Can you work these out from the drawing? Everything is in mm from the part's minimum corner. A direction names the side the tool comes from. Round coordinates to 2 decimals unless told otherwise and drop trailing zeros. Loops run counter-clockwise (first coordinate to the right, second up) from the corner with the lowest first, then second, coordinate; pieces in that order, holes last. Notation, with made-up numbers: M 10,1.5 L 51,1.5 A14 cw 51,9.5 Z; hole C 79,65.5 d8. An arc over 180 degrees is marked long. Use a Markdown table: item, result.
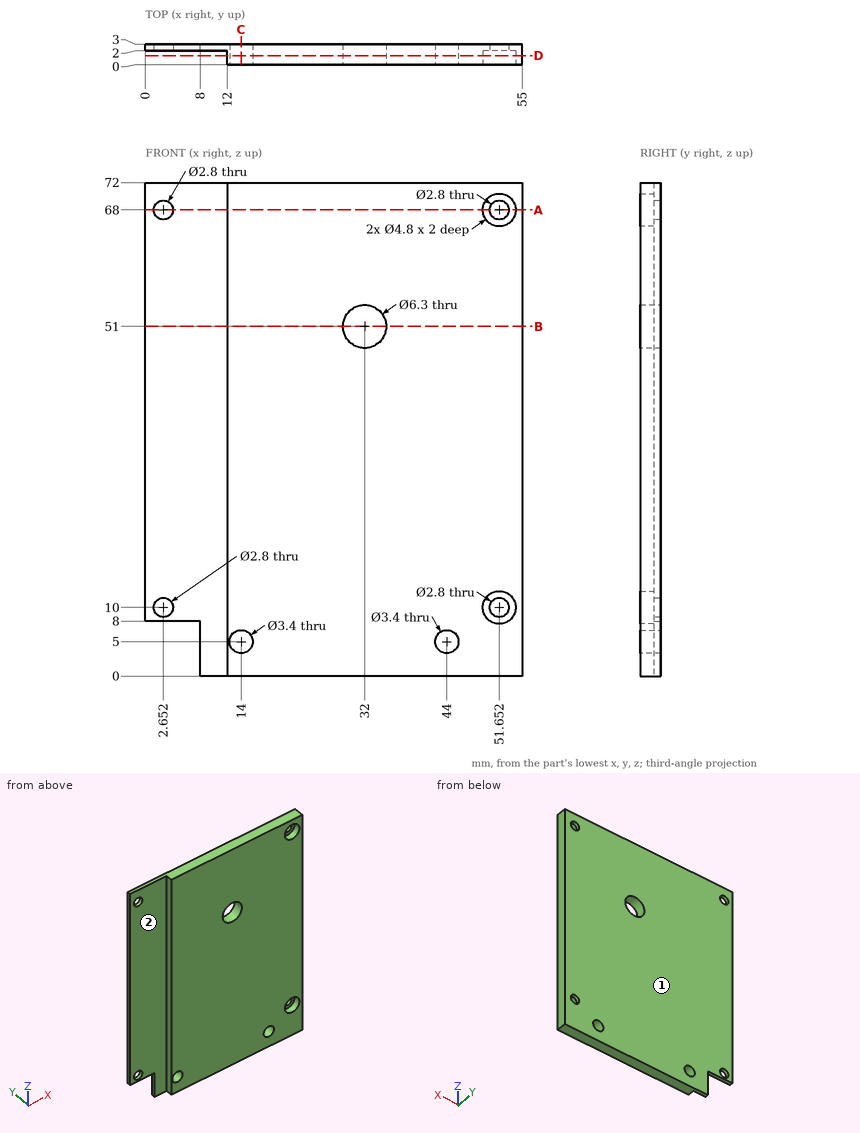
1. Imagine slicing it at A-A, the plane z = 68. Write out the boundary of the cut face in (x, y).
Answer sheet:
| item | result |
|---|---|
| outline | M 0,2 L 1.25,2 L 1.25,3 L 0,3 Z; M 4.05,2 L 12,2 L 12,0 L 49.25,0 L 49.25,2 L 50.25,2 L 50.25,3 L 4.05,3 Z; M 53.05,2 L 54.05,2 L 54.05,0 L 55,0 L 55,3 L 53.05,3 Z |
2. Imagine slicing it at B-B, the plane z = 51. Write out the boundary of the cut face in (x, y), then the cut area to 3 significant figures.
Answer sheet:
| item | result |
|---|---|
| outline | M 0,2 L 12,2 L 12,0 L 28.85,0 L 28.85,3 L 0,3 Z; M 35.15,0 L 55,0 L 55,3 L 35.15,3 Z |
| area | 122 mm2 |
3. Imagine slicing it at C-C, the plane x = 14. Write out the boundary of the cut face in (y, z), then the cut area to 3 significant figures.
Answer sheet:
| item | result |
|---|---|
| outline | M 0,0 L 3,0 L 3,3.3 L 0,3.3 Z; M 0,6.7 L 3,6.7 L 3,72 L 0,72 Z |
| area | 206 mm2 |
4. I need wall thicknesses on probe 1 along X at (y, z) = (2.5, 68); probe 2 along Y at (x, z) = (8.5, 6.5); probe 3 along X at (y, z) = (1, 35). Which ranges of each line are inside material? Lowest first, please. Write a range as from..to.
Answer sheet:
| item | result |
|---|---|
| probe 1 | 0..1.25, 4.05..50.25, 53.05..55 |
| probe 2 | 2..3 |
| probe 3 | 12..55 |
5. Imagine slicing it at D-D, the plane y = 1.3. Write out the boundary of the cut face in (x, z).
Answer sheet:
| item | result |
|---|---|
| outline | M 12,0 L 55,0 L 55,72 L 12,72 Z; hole C 14,5 d3.4; hole C 32,51 d6.3; hole C 44,5 d3.4; hole C 51.65,10 d4.8; hole C 51.65,68 d4.8 |
6. Which directions (+Z, -Z, +X, -X, +Y, -Y) give clear straight access to the entire face, cutting with the end or side of a thin tool? Please do the marked faces 1 and 2.
Answer sheet:
| item | result |
|---|---|
| face 1 | +Z, -Z, +X, -X, +Y |
| face 2 | +Z, -Z, -X, -Y |
7. For pin 1 Ø2.5 at (x, z) = (51, 11) entering from -Y; pin 2 Ø3 at (x, z) = (2.65, 10) entering from -Y; pin 3 Ø1.7 at (x, z) = (51.65, 10) entering from +Y, each with a flat end and sliding along its axis, tell me the tip position at first contact or that it passes through.
Answer sheet:
| item | result |
|---|---|
| pin 1 | y = 0 |
| pin 2 | y = 2 |
| pin 3 | through |
